The listing builds one solid part. Answer for the finished solid, in the listing's coordinates (mm). A direction names the side the tool comes from. Round coordinates to 2 decimals unless told otherwise and drop trailing zeros. Write each loop counter-clockwise with the first axis right and the second up, starting at its lowest first coordinate (ties: lowest second). Pieces come first, ordered by that corner, then holes.
(1) A cutting plane is placed at A-A, the plane x = 36.5. Give the vertices of the cut face in (y, z), and give its area (3 significant figures).
(2) A cutting plane is placed at B-B, the plane y = 2.5. Give the vertices of the cut face in (x, z), and give its area (3 significant figures).
(3) The mould has two halves that part along Y. Classify faces 1 (the face through (19, 16, 0)), 2 (the face through (19, 30.59, -1)), 3 (the face through (19, 0, -1)), 4 (the face through (3, 27, -2)): +Y half, -Y half, draft (parallel to the pull), parting line (faces both ways), or undercut.
(4) For faces 5 (the face through (34.502, 2.588, -0.986)), 6 (the face through (0, 15, -1)), determine the directions among +Z, -Z, +X, -X, +Y, -Y from which every point of the face is accessible in a straight line to the end or side of a thin tool.
(5) Find the intervals of material crossed by probe 1 along Y at (x, z) = (2.5, -2.25); probe 2 along Y at (x, z) = (36.5, -1.35); probe 3 along X at (y, z) = (27, -0.75), in increasing order.
(6) Each of these flat-tipped pins is pushed along its axis until it touches: pin 1 Ø3 at (x, y) = (36.5, 28.09) entering from +Z; pin 2 Ø4.5 at (x, y) = (3, 3) entering from +Z; pin 3 Ø1.6 at (x, y) = (36.5, 28.09) entering from -Z. Where does it stop, or does it pass through?
(7) A cutting plane is placed at C-C, the plane z = -1.4. Give the vertices of the cut face in (x, y), and give its area (3 significant figures).
from build123d import *

# Parameters (mm, degrees)
SKETCH_1_W                   = 39
SKETCH_1_H                   = 30.59
EXTRUDE_1_DEPTH              = 2.5
SKETCH_2_W                   = 5
SKETCH_2_H                   = 5
EXTRUDE_2_DEPTH              = 2.5
HOLE_WIZARD_M2_8_D           = 2
HOLE_WIZARD_M2_8_DEPTH       = 3
HOLE_WIZARD_M2_8_CBORE_D     = 4
HOLE_WIZARD_M2_8_CBORE_DEPTH = 2
HOLE_WIZARD_M2_7_D           = 2
HOLE_WIZARD_M2_7_DEPTH       = 3
HOLE_WIZARD_M2_7_CBORE_D     = 4
HOLE_WIZARD_M2_7_CBORE_DEPTH = 2


with BuildPart() as part:
    # 草图1 → 凸台-拉伸1 (new body)
    with BuildSketch(Plane.XY):
        with Locations((19.5, 15.295)):
            Rectangle(SKETCH_1_W, SKETCH_1_H)
    extrude(amount=-EXTRUDE_1_DEPTH)

    # 草图2 → 凸台-拉伸2 (add)
    with BuildSketch(Plane.XY):
        with Locations((2.5, 2.5)):
            Rectangle(SKETCH_2_W, SKETCH_2_H)
        with Locations((36.5, 28.09)):
            Rectangle(SKETCH_2_W, SKETCH_2_H)
    extrude(amount=-EXTRUDE_2_DEPTH)

    # M2 六角头螺栓的柱形沉头孔8
    with Locations(Plane(origin=(2.5, 2.5, 0), x_dir=(1, 0, 0), z_dir=(0, 0, 1))):
        with Locations((0, 0), (34, 25.59)):
            CounterBoreHole(HOLE_WIZARD_M2_8_D / 2, HOLE_WIZARD_M2_8_CBORE_D / 2, HOLE_WIZARD_M2_8_CBORE_DEPTH, depth=HOLE_WIZARD_M2_8_DEPTH)

    # M2 六角头螺栓的柱形沉头孔7
    with Locations(Plane.XY):
        with Locations((2.5, 28.09), (36.5, 2.5)):
            CounterBoreHole(HOLE_WIZARD_M2_7_D / 2, HOLE_WIZARD_M2_7_CBORE_D / 2, HOLE_WIZARD_M2_7_CBORE_DEPTH, depth=HOLE_WIZARD_M2_7_DEPTH)


solid = part.part
Solutions:
1. outline: (0, -2.5) - (1.5, -2.5) - (1.5, -2) - (0.5, -2) - (0.5, 0) - (0, 0) - close; (3.5, -2.5) - (27.09, -2.5) - (27.09, -2) - (26.09, -2) - (26.09, 0) - (4.5, 0) - (4.5, -2) - (3.5, -2) - close; (29.09, -2.5) - (30.59, -2.5) - (30.59, 0) - (30.09, 0) - (30.09, -2) - (29.09, -2) - close
1. area: 58.5 mm2
2. outline: (0, -2.5) - (1.5, -2.5) - (1.5, -2) - (0.5, -2) - (0.5, 0) - (0, 0) - close; (3.5, -2.5) - (35.5, -2.5) - (35.5, -2) - (34.5, -2) - (34.5, 0) - (4.5, 0) - (4.5, -2) - (3.5, -2) - close; (37.5, -2.5) - (39, -2.5) - (39, 0) - (38.5, 0) - (38.5, -2) - (37.5, -2) - close
2. area: 79.5 mm2
3. face 1: draft
3. face 2: +Y half
3. face 3: -Y half
3. face 4: undercut
4. face 5: +Z
4. face 6: +Z, -Z, -X, +Y, -Y
5. probe 1: y = 0 to 1.5, 3.5 to 27.09, 29.09 to 30.59
5. probe 2: y = 0 to 0.5, 4.5 to 26.09, 30.09 to 30.59
5. probe 3: x = 0 to 0.82, 4.18 to 34.82, 38.18 to 39
6. pin 1: stops at z = -2
6. pin 2: stops at z = 0
6. pin 3: passes through
7. outline: (0, 0) - (39, 0) - (39, 30.59) - (0, 30.59) - close; hole circle Ø4 at (2.5, 2.5); hole circle Ø4 at (2.5, 28.09); hole circle Ø4 at (36.5, 2.5); hole circle Ø4 at (36.5, 28.09)
7. area: 1,140 mm2
